```python
from build123d import *

# Parameters (mm, degrees)
BOSS_EXTRUDE1_START      = -1
SKETCH1_W                = 1.7
SKETCH1_H                = 89.2
BOSS_EXTRUDE1_DEPTH      = 9.2
SKETCH4_W                = 33.7
SKETCH4_H                = 11.6
BOSS_EXTRUDE3_DEPTH      = 9.2
SERVO_HOLDER_DEPTH       = 1
SERVO_HOLDER_DEPTH_BACK  = 9.2
SKETCH3_W                = 14
SKETCH3_H                = 7
SKETCH3_R                = 1
SKETCH37_W               = 20
SKETCH37_H               = 7
BOSS_EXTRUDE19_DEPTH     = 10.2
CUT_EXTRUDE10_DEPTH      = 93.482268571
CUT_EXTRUDE10_DEPTH_BACK = 93.482268571
SKETCH29_W               = 34.409909993
SKETCH29_H               = 5.977389624
BOSS_EXTRUDE13_START     = 2
SKETCH30_W               = 34
SKETCH30_H               = 38
SKETCH30_R               = 1.6
BOSS_EXTRUDE13_DEPTH     = 6.5
SKETCH41_W               = 17.288461538
SKETCH41_H               = 9.2
CUT_EXTRUDE14_DEPTH      = 15
BOSS_EXTRUDE14_START     = -38
SKETCH32_R               = 1.45
SKETCH32_R_2             = 5
BOSS_EXTRUDE14_DEPTH     = 8.8
BOSS_EXTRUDE16_DEPTH     = 3
BOSS_EXTRUDE17_DEPTH     = 3
BOSS_EXTRUDE18_START     = -9.2
BOSS_EXTRUDE18_DEPTH     = 9.2
SKETCH39_W               = 1.7
SKETCH39_H               = 41.2
BOSS_EXTRUDE20_DEPTH     = 9.2
CUT_EXTRUDE13_DEPTH      = 17.5
CHAMFER2_SIZE            = 0.6
CHAMFER2_SIZE_2          = 1.039230485
CHAMFER3_SIZE            = 3
FILLET10_R               = 6
CUT_EXTRUDE15_DEPTH      = 10
CHAMFER4_SIZE            = 2.5
CUT_EXTRUDE16_DEPTH      = 10
FILLET11_R               = 0.8
SKETCH44_W               = 59.192885725
SKETCH44_H               = 45.417181718
CUT_EXTRUDE17_DEPTH      = 87.948983376


with BuildPart() as part:
    # Sketch1 → Boss-Extrude1 (new body)
    with BuildSketch(Plane(origin=(0, 0, 0), x_dir=(1, 0, 0), z_dir=(0, 1, 0)).offset(BOSS_EXTRUDE1_START)):
        with Locations((-20.85, 25.311538462)):
            Rectangle(SKETCH1_W, SKETCH1_H)
    extrude(amount=-BOSS_EXTRUDE1_DEPTH)

    # Sketch4 → Boss-Extrude3 (add)
    with BuildSketch(Plane.XZ.offset(10.2)):
        with Locations((-4.85, -64.111538462)):
            Rectangle(SKETCH4_W, SKETCH4_H)
    extrude(amount=-BOSS_EXTRUDE3_DEPTH)

    # Sketch3 → Servo Holder (add, two sides: drawn at the far end of the back side and taken through both)
    # profile 1 of 2: a face of its own
    with BuildSketch(Plane.XZ.offset(10.2).offset(-SERVO_HOLDER_DEPTH_BACK)):
        with Locations((-14.7, -55.411538462)):
            Rectangle(SKETCH3_W, SKETCH3_H)
        with Locations(Location((-14, -54.311538462, 0), (0, 0, 270))):
            Circle(SKETCH3_R, mode=Mode.SUBTRACT)
    # profile 2 of 2: a face of its own
    with BuildSketch(Plane.XZ.offset(10.2).offset(-SERVO_HOLDER_DEPTH_BACK)):
        with Locations((-14.7, -25.211538462)):
            Rectangle(SKETCH3_W, SKETCH3_H)
        with Locations(Location((-14, -26.311538462, 0), (0, 0, 90))):
            Circle(SKETCH3_R, mode=Mode.SUBTRACT)
    extrude(amount=SERVO_HOLDER_DEPTH + SERVO_HOLDER_DEPTH_BACK)

    # Sketch37 → Boss-Extrude19 (add)
    with BuildSketch(Plane(origin=(0, -1, 0), x_dir=(1, 0, 0), z_dir=(0, 1, 0))):
        with Locations((2.3, 25.211538462)):
            Rectangle(SKETCH37_W, SKETCH37_H)
    extrude(amount=-BOSS_EXTRUDE19_DEPTH)

    # Sketch29 → Cut-Extrude10 (cut, two sides: drawn at the far end of the back side and taken through both)
    with BuildSketch(Plane(origin=(0, 0, -69.911538462), x_dir=(-1, 0, 0), z_dir=(0, 0, -1)).offset(-CUT_EXTRUDE10_DEPTH_BACK)):
        with Locations((4.495045004, -13.188694812)):
            Rectangle(SKETCH29_W, SKETCH29_H)
    extrude(amount=CUT_EXTRUDE10_DEPTH + CUT_EXTRUDE10_DEPTH_BACK, mode=Mode.SUBTRACT)


with BuildPart() as body_2:
    # Sketch30 → Boss-Extrude13 (new body)
    with BuildSketch(Plane.XY.offset(BOSS_EXTRUDE13_START)):
        with Locations((-4.7, -20)):
            Rectangle(SKETCH30_W, SKETCH30_H)
        with Locations(Location((5.3, -34, 0), (0, 0, 180))):
            Circle(SKETCH30_R, mode=Mode.SUBTRACT)
        with Locations(Location((5.3, -19, 0), (0, 0, 180))):
            Circle(SKETCH30_R, mode=Mode.SUBTRACT)
        with Locations(Location((-14.7, -34, 0), (0, 0, 180))):
            Circle(SKETCH30_R, mode=Mode.SUBTRACT)
        with Locations(Location((-14.7, -19, 0), (0, 0, 180))):
            Circle(SKETCH30_R, mode=Mode.SUBTRACT)
    extrude(amount=BOSS_EXTRUDE13_DEPTH)


with BuildPart() as cut_extrude14_tool:
    # Sketch41 → Cut-Extrude14 (new body)
    with BuildSketch(Plane(origin=(-20, 0, 0), x_dir=(0, 0, -1), z_dir=(1, 0, 0))):
        with Locations((-10.644230769, -5.6)):
            Rectangle(SKETCH41_W, SKETCH41_H)
    extrude(amount=-CUT_EXTRUDE14_DEPTH)


with BuildPart() as part_1:
    add(part.part)

    # Cut-Extrude14: cut by cut_extrude14_tool
    add(cut_extrude14_tool.part, mode=Mode.SUBTRACT)



with BuildPart() as body_2_1:
    add(body_2.part)

    # Cut-Extrude14: cut by cut_extrude14_tool
    add(cut_extrude14_tool.part, mode=Mode.SUBTRACT)

    # Sketch32 → Boss-Extrude14 (add)
    with BuildSketch(Plane.XZ.offset(39).offset(BOSS_EXTRUDE14_START)):
        with BuildLine():
            ThreePointArc((11.872921748, 2), (25.925390485, -3.535644523), (35.05, 8.5))
            ThreePointArc((35.05, 8.5), (22.55, 21), (10.05, 8.5))
            Line((10.05, 8.5), (12.3, 8.5))
            Line((12.3, 8.5), (12.3, 2))
            Line((12.3, 2), (11.872921748, 2))
        make_face()
        with Locations(Location((15.25884337, 2.409923235, 0), (0, 0, 180))):
            Circle(SKETCH32_R, mode=Mode.SUBTRACT)
        with Locations(Location((28.640076765, 1.20884337, 0), (0, 0, 180))):
            Circle(SKETCH32_R, mode=Mode.SUBTRACT)
        with Locations(Location((16.459923235, 15.79115663, 0), (0, 0, 180))):
            Circle(SKETCH32_R, mode=Mode.SUBTRACT)
        with Locations(Location((22.55, 8.5, 0), (0, 0, 180))):
            Circle(SKETCH32_R_2, mode=Mode.SUBTRACT)
        with Locations(Location((29.84115663, 14.590076765, 0), (0, 0, 180))):
            Circle(SKETCH32_R, mode=Mode.SUBTRACT)
    extrude(amount=BOSS_EXTRUDE14_DEPTH)


with BuildPart() as part_2:
    add(part_1.part)

    add(body_2_1.part)  # Boss-Extrude16 merges body 2
    # Sketch34 → Boss-Extrude16 (add)
    with BuildSketch(Plane.ZY.offset(21.7)):
        Polygon((-21.711538462, -1), (-21.711538462, -9.8), (2, -39), (8.5, -39), (8.5, -1), align=None)
    extrude(amount=-BOSS_EXTRUDE16_DEPTH)

    # Sketch35 → Boss-Extrude17 (add)
    with BuildSketch(Plane(origin=(12.3, 0, 0), x_dir=(0, 0, -1), z_dir=(1, 0, 0))):
        Polygon((-2, -1), (21.711538462, -1), (21.711538462, -9.8), (-2, -39), (-8.5, -39), (-8.5, -9.8), (-8.5, -1), align=None)
    extrude(amount=-BOSS_EXTRUDE17_DEPTH)

    # Sketch36 → Boss-Extrude18 (add)
    with BuildSketch(Plane.XZ.offset(10.2).offset(BOSS_EXTRUDE18_START)):
        Polygon((12.3, -10.579162849), (16.63422252, -2.511520186), (12.3, 1.345455989), align=None)
    extrude(amount=BOSS_EXTRUDE18_DEPTH)

    # Sketch39 → Boss-Extrude20 (add)
    with BuildSketch(Plane(origin=(0, -1, 0), x_dir=(1, 0, 0), z_dir=(0, 1, 0))):
        with Locations((11.45, 49.311538462)):
            Rectangle(SKETCH39_W, SKETCH39_H)
    extrude(amount=-BOSS_EXTRUDE20_DEPTH)

    # Sketch40 → Cut-Extrude13 (cut)
    with BuildSketch(Plane(origin=(12.3, 0, 0), x_dir=(0, 0, -1), z_dir=(1, 0, 0))):
        Polygon((64.111538462, -1), (60.611538462, -1), (60.611538462, -2.2), (59.611538462, -2.2), (59.611538462, -6.2), (64.111538462, -6.2), align=None)
        Polygon((67.611538462, -1), (64.111538462, -1), (64.111538462, -6.2), (68.611538462, -6.2), (68.611538462, -2.2), (67.611538462, -2.2), align=None)
    extrude(amount=-CUT_EXTRUDE13_DEPTH, mode=Mode.SUBTRACT)

    # Chamfer2
    # the kernel refuses this chamfer: 1.039230485, 0.6 mm, written as the material it takes off along each edge
    with BuildSketch(Plane(origin=(14.988578382, -2.2, -67.611538462), x_dir=(0, 0.9983227437537925, 0.05789386240267319), z_dir=(-1, 0, 0))) as chamfer2_piece_1_section:
        Polygon((CHAMFER2_SIZE * 0.998322743754, CHAMFER2_SIZE * 0.0578938624027), (-CHAMFER2_SIZE_2 * 0.0578938623771, CHAMFER2_SIZE_2 * 0.998322743313), (0, 0), align=None)
    chamfer2_piece_1 = extrude(amount=20.188578382, mode=Mode.PRIVATE)
    chamfer2_piece_1 = split(chamfer2_piece_1, bisect_by=Plane(origin=(4.894289191, -2.005782009, -68.611538462), z_dir=(0, 0, 1)), keep=Keep.TOP, mode=Mode.PRIVATE)
    add(chamfer2_piece_1, mode=Mode.SUBTRACT)
    with BuildSketch(Plane(origin=(14.988578382, -2.2, -60.611538462), x_dir=(0, 0.9983227437537925, -0.05789386240267317), z_dir=(-1, 0, 0))) as chamfer2_piece_2_section:
        Polygon((CHAMFER2_SIZE * 0.998322743754, -CHAMFER2_SIZE * 0.0578938624027), (-CHAMFER2_SIZE_2 * 0.0578938623771, -CHAMFER2_SIZE_2 * 0.998322743313), (0, 0), align=None)
    chamfer2_piece_2 = extrude(amount=20.188578382, mode=Mode.PRIVATE)
    chamfer2_piece_2 = split(chamfer2_piece_2, bisect_by=Plane(origin=(4.894289191, -2.005782009, -59.611538462), z_dir=(0, 0, -1)), keep=Keep.TOP, mode=Mode.PRIVATE)
    add(chamfer2_piece_2, mode=Mode.SUBTRACT)

    # Chamfer3
    chamfer3_edges = [part_2.edges().sort_by_distance(p)[0] for p in [
        (10.6, -5.6, -58.311538462),
        (10.6, -5.6, -28.711538462),
    ]]
    chamfer(chamfer3_edges, length=CHAMFER3_SIZE)

    # Fillet10
    fillet10_edges = [part_2.edges().sort_by_distance(p)[0] for p in [
        (16.63422252, -5.4, -2.511520186),
        (12.3, -5.6, -10.579162849),
    ]]
    fillet(fillet10_edges, radius=FILLET10_R)

    # Sketch42 → Cut-Extrude15 (cut)
    with BuildSketch(Plane.XY.offset(8.5)):
        with BuildLine():
            Line((-1.1, -1), (-1.1, -10.6))
            ThreePointArc((-1.1, -10.6), (-4.7, -14.2), (-8.3, -10.6))
            Line((-8.3, -10.6), (-8.3, -1))
            Line((-8.3, -1), (-1.1, -1))
        make_face()
    extrude(amount=-CUT_EXTRUDE15_DEPTH, mode=Mode.SUBTRACT)

    # Chamfer4
    chamfer4_edges = [part_2.edges().sort_by_distance(p)[0] for p in [
        (-7.7, -5.6, -58.311538462),
    ]]
    chamfer(chamfer4_edges, length=CHAMFER4_SIZE)

    # Sketch43 → Cut-Extrude16 (cut)
    with BuildSketch(Plane(origin=(0, -1, 0), x_dir=(1, 0, 0), z_dir=(0, 1, 0))):
        Polygon((-5.2, 58.311538462), (-11.6, 51.911538462), (-5.2, 51.911538462), align=None)
    extrude(amount=-CUT_EXTRUDE16_DEPTH, mode=Mode.SUBTRACT)

    # Fillet11
    fillet11_edges = [part_2.edges().sort_by_distance(p)[0] for p in [
        (-20, -5.6, -28.711538462),
        (-20, -5.6, -51.911538462),
        (10.6, -5.6, -55.311538462),
        (10.6, -5.6, -31.711538462),
        (7.6, -5.6, -28.711538462),
        (7.6, -5.6, -58.311538462),
        (-5.2, -5.6, -58.311538462),
        (-11.6, -5.6, -51.911538462),
    ]]
    fillet(fillet11_edges, radius=FILLET11_R)

    # Sketch44 → Cut-Extrude17 (cut, through all)
    with BuildSketch(Plane(origin=(0, -1, 0), x_dir=(1, 0, 0), z_dir=(0, 1, 0))):
        with Locations((7.896442862, -0.997052397)):
            Rectangle(SKETCH44_W, SKETCH44_H)
    extrude(amount=-CUT_EXTRUDE17_DEPTH, mode=Mode.SUBTRACT)


solid = part_2.part
```
Could you check a few things on this model? Use its own coordinates, in mm. A direction names the side the tool comes from. Give positions to 0.01 mm unless a question says otherwise; leave off trailing zeros. Write each loop counter-clockwise with the first axis right and the second up, starting at its lowest first coordinate (ties: lowest second). Pieces come first, ordered by that corner, then holes. Notation, with made-up numbers: (-3.5, -9.75) - (15.5, -9.75) arc R23 cw to (15.5, 9.25) - close; hole circle Ø9 at (-23, 10.25). An arc over 180 degrees is marked (long way). One line per item, written item: value. Start each with the question number.
Item 1: Please list where these lines run through material, in increasing order: line 1 (Z direction, x = -14, y = -5.75); line 2 (Z direction, x = -3.5, y = -4); line 3 (X direction, y = -4.5, z = -36). Write a range as from..to.
Item 2: If we mould it in two halves opening along X, with no side actions, what happens to faces 1 (the face through (-13.024, -5.536, -26.528)), 2 (the face through (12.3, -6, -45)), 3 (the face through (-5, -6, -21.712))? For each: +X half, -X half, draft (parallel to the pull), parting line (faces both ways), or undercut.
Item 3: Imagine slicing it at C-C, the plane y = -2.75. List the corners of the cut face in (x, z) for me, and give its area (3 significant figures).
Item 4: Imagine slicing it at A-A, the plane z = -49. List the corners of the cut face in (x, y) for me, and give its area (3 significant figures).
Item 5: Which directions (+Z, -Z, +X, -X, +Y, -Y) give clear straight access to the entire face, cutting with the end or side of a thin tool? Please do faces 4 (the face through (-5, -6, -69.912)), 5 (the face through (9.08, -5.54, -30.19)), 6 (the face through (3.672, -1.885, -60.119)).
Item 6: I'm going to push flat-ended pins straight in: pin 1 (2.5 mm diameter, centred on x = 4.5, z = -65.5, fed in from +Y); pin 2 (2.5 mm diameter, centred on y = -3, z = -65.5, fed in from +X). Where does each tip first touch, or does it pass through?
Item 7: Imagine slicing it at D-D, the plane x = 0. List the corners of the cut face in (y, z) for me, and give its area (3 significant figures).
Item 8: Imagine slicing it at B-B, the plane x = -12.5. List the corners of the cut face in (y, z) for me.
Geometry says:
1. line 1: -69.91..-55.31, -53.31..-51.91, -28.71..-27.31, -25.31..-21.71
1. line 2: -69.91..-68.61, -59.61..-58.31, -28.71..-21.71
1. line 3: -21.7..-20, 10.6..12.3
2. face 1: undercut
2. face 2: +X half
2. face 3: draft
3. outline: (-21.7, -69.91) - (12.3, -69.91) - (12.3, -68.61) - (-5.2, -68.61) - (-5.2, -59.61) - (12.3, -59.61) - (12.3, -21.71) - (-21.7, -21.71) - close; hole (-20, -51.11) arc R0.8 ccw to (-19.2, -51.91) - (-11.93, -51.91) arc R0.8 cw to (-11.37, -52.15) - (-5.43, -58.08) arc R0.8 ccw to (-4.87, -58.31) - (7.27, -58.31) arc R0.8 ccw to (7.83, -58.08) - (10.37, -55.55) arc R0.8 ccw to (10.6, -54.98) - (10.6, -32.04) arc R0.8 ccw to (10.37, -31.48) - (7.83, -28.95) arc R0.8 ccw to (7.27, -28.71) - (-19.2, -28.71) arc R0.8 ccw to (-20, -29.51) - close; hole circle Ø2 at (-14, -54.31); hole circle Ø2 at (-14, -26.31)
3. area: 653 mm^2
4. outline: (-21.7, -10.2) - (-20, -10.2) - (-20, -1) - (-21.7, -1) - close; (10.6, -10.2) - (12.3, -10.2) - (12.3, -1) - (10.6, -1) - close
4. area: 31.3 mm^2
5. face 4: -Z, +X, -X, +Y, -Y
5. face 5: +Y, -Y
5. face 6: +X
6. pin 1: y = -6.2
6. pin 2: x = -5.2
7. outline: (-10.2, -69.91) - (-1, -69.91) - (-1, -67.61) - (-1.6, -67.61) - (-2.18, -68.61) - (-6.2, -68.61) - (-6.2, -59.61) - (-2.18, -59.61) - (-1.6, -60.61) - (-1, -60.61) - (-1, -58.31) - (-10.2, -58.31) - close; (-10.2, -28.71) - (-1, -28.71) - (-1, -21.71) - (-10.2, -21.71) - close
7. area: 126 mm^2
8. outline: (-10.2, -69.91) - (-1, -69.91) - (-1, -51.91) - (-10.2, -51.91) - close; (-10.2, -28.71) - (-1, -28.71) - (-1, -21.71) - (-10.2, -21.71) - close
